Answer from the drawing. Dimensions are ordinates in mm from the lowest x, y and z of the part. A direction names the side the tool comes from. Give positions to 0.01 mm unless a question says otherwise; leave off trailing zeros. Order: outer loops, then holes, each group sorted by start corner. A loop starts at its lowest first (then second) coordinate and runs counter-clockwise, first axis right, second up. Notation, with made-up numbers: (58, 25.5) -> (95, 25.5) arc R22 cw to (95, 60.5) -> close; hole circle Ø1 at (66, 50.25). An arc over 180 degrees is marked (long way). Answer as CSV lines item,"result". Start each with the question number.
1) Straight lines are drawn through the part: L1, parallel to Y at x = 6, z = 9; L2, parallel to Z at x = 6.25, y = 15.5; L3, parallel to Y at x = 6, z = 13.5. For each, find the intervals that lie inside material, in ascending order. Write a range as from..to.
2) Find section C-C (z = 10.75). Determine the outline of the cut face in (x, y).
3) Find section B-B (z = 17). Determine the outline of the cut face in (x, y), and give its area (3 significant figures).
4) The mould has two halves that part along X. Classify the marked faces 1, 2, 3 and 4: +X half, -X half, draft (parallel to the pull), parting line (faces both ways), or undercut.
5) For the marked faces 5 and 6, determine the directions among +Z, -Z, +X, -X, +Y, -Y from which every point of the face is accessible in a straight line to the end or side of a thin tool.
6) Flat-ended cylindrical pins translate along their axes: pin 1 Ø1 at (x, z) = (2.5, 16) entering from +Y; pin 2 Ø1.5 at (y, z) = (3.5, 9) entering from -X; pin 3 Ø4.5 at (x, y) = (6, 6) entering from -Z. Find the tip coordinate at first contact, or state that the pin passes through.
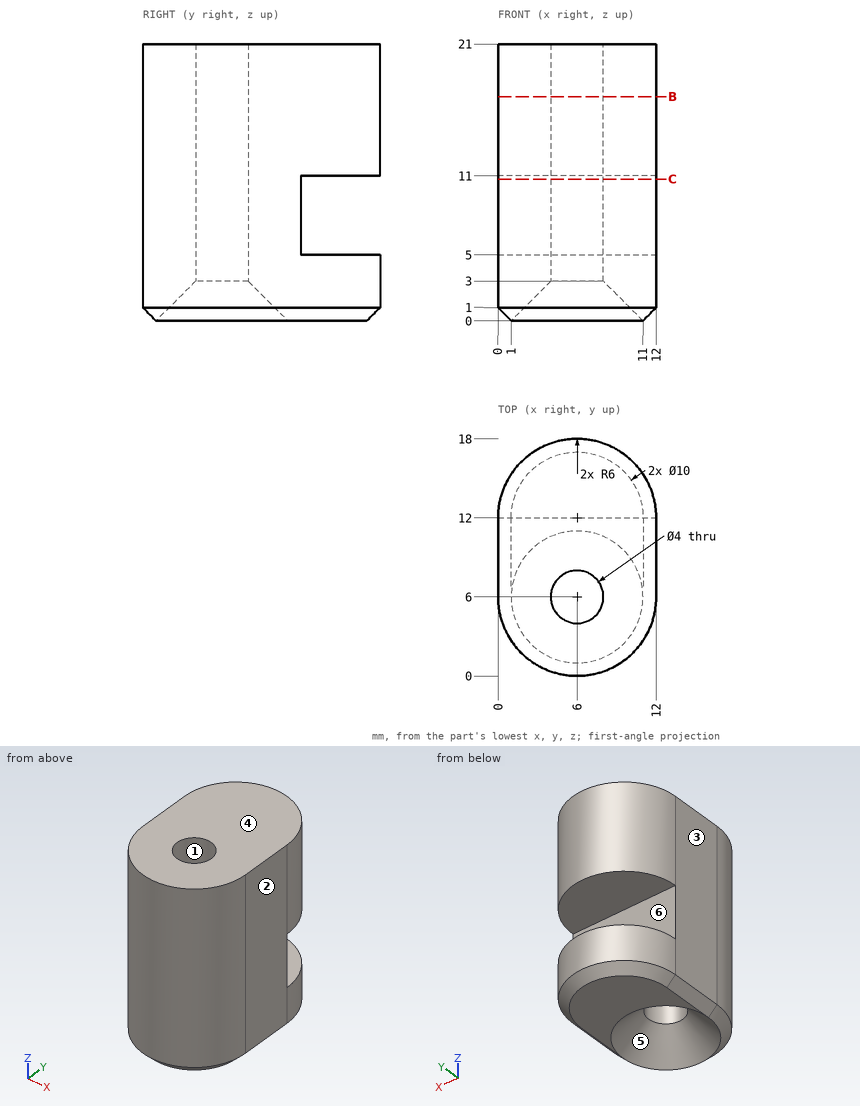
Findings below:
1,L1,"0..4, 8..12"
1,L2,"0..5, 11..21"
1,L3,"0..4, 8..18"
2,outline,"(0, 6) arc R6 ccw to (12, 6) -> (12, 12) -> (0, 12) -> close; hole circle Ø4 at (6, 6)"
3,outline,"(0, 6) arc R6 ccw to (12, 6) -> (12, 12) arc R6 ccw to (0, 12) -> close; hole circle Ø4 at (6, 6)"
3,area,"173 mm²"
4,face 1,"undercut"
4,face 2,"+X half"
4,face 3,"-X half"
4,face 4,"draft"
5,face 5,"-Z"
5,face 6,"+X, -X, +Y"
6,pin 1,"y = 17.2"
6,pin 2,"x = 0.26"
6,pin 3,"z = 2.75"
